Autodesk Fusion 360 part; units mm, degrees
sketch "Sketch1" plane through (0, 0, 0) normal (0, 0, 1) x (1, 0, 0)
  line L0 (0, 0) -> (-25, 0)
  line L1 (-25, 0) -> (-25, 25)
  line L2 (-25, 25) -> (0, 25)
  line L3 (0, 25) -> (0, 0)
  dimension "d1" = 25
  dimension "d2" = 25
extrude "Extrude1" add sketch "Sketch1" along normal blind 5
sketch "Sketch2" plane through (0, 0, 5) normal (0, 0, 1) x (-1, 0, 0)
  line L0 (0, -25) -> (25, -25)
  line L1 (25, -25) -> (25, 0)
  line L2 (25, 0) -> (0, 0)
  line L3 (0, 0) -> (0, -25)
  line L4 (12.5, -25) -> (12.5, 0)
  line L5 (12.5, -12.5) -> (0, -12.5)
  circle A0 centre (12.5, -12.5) radius 10
  dimension "d5" = 20
extrude "Extrude2" add sketch "Sketch2" along normal blind 5 contours L4 L5 A0 | L4 A0 | L4 L5 A0
sketch "Sketch3" plane through (0, 0, 10) normal (0, 0, 1) x (-1, 0, 0)
  circle A0 centre (12.5, -12.5) radius 10
  line L0 (11, -17) -> (14, -17)
  line L1 (14, -17) -> (14, -23)
  line L2 (14, -23) -> (11, -23)
  line L3 (11, -23) -> (11, -17)
extrude "Extrude3" cut sketch "Sketch3" against normal blind 3 contours A0 L0 L1 L3 picked at (12.6672, -18.8291)
Can you work these out from the model? Positions are in its coordinate system, mm. A direction names the side the tool comes from. Give positions to 0.01 mm unless a question says otherwise; leave off trailing zeros. Loops run counter-clockwise (first coordinate to the right, second up) from the corner with the lowest first, then second, coordinate; pieces in that order, holes last. Notation, with made-up numbers: M 56,88.25 L 77,88.25 A35 cw 77,126.25 Z; hole C -11.5,-35 d2. An arc over 180 degrees is marked long. Answer in a Markdown table with one row per item.
1. Suppose I cut it at B-B on x = -5.5. Write out the boundary of the cut face in (y, z).
Taken from the geometry:
| item | result |
|---|---|
| outline | M 0,0 L 25,0 L 25,5 L 19.64,5 L 19.64,10 L 5.36,10 L 5.36,5 L 0,5 Z |
2. Suppose I cut it at D-D on x = -12.5. Write out the boundary of the cut face in (y, z), plus the area to 4 significant figures.
Taken from the geometry:
| item | result |
|---|---|
| outline | M 0,0 L 25,0 L 25,5 L 22.5,5 L 22.5,7 L 17,7 L 17,10 L 2.5,10 L 2.5,5 L 0,5 Z |
| area | 208.5 mm² |
3. If I drill on line 1 along Z through (x, y) = (-19.25, 23.25); line 2 along X through (y, z) = (12.75, 8); line 3 along Y through (x, z) = (-18.5, 8), over which ranges is the centre line in solid material (lowest first)?
Taken from the geometry:
| item | result |
|---|---|
| line 1 | z = 0 to 5 |
| line 2 | x = -22.5 to -2.5 |
| line 3 | y = 4.5 to 20.5 |
4. Which directions (+Z, -Z, +X, -X, +Y, -Y) give clear straight access to the entire face, cutting with the end or side of a thin tool? Please do faces 5 (the flat face through (-13, 25, 2)), 6 (the flat face through (-12, 20, 7)), 7 (the flat face through (-21, 18.2, 5)).
Taken from the geometry:
| item | result |
|---|---|
| face 5 | +Z, -Z, +X, -X, +Y |
| face 6 | +Z, +Y |
| face 7 | +Z |
5. Suppose I cut it at C-C on z = 9.25. Write out the boundary of the cut face in (x, y), plus the area to 3 significant figures.
Taken from the geometry:
| item | result |
|---|---|
| outline | M -14,17 L -14,22.39 A10 ccw long -11,22.39 L -11,17 Z |
| area | 298 mm² |
6. Suppose I cut it at A-A on y = 12.5. Write out the boundary of the cut face in (x, z).
Taken from the geometry:
| item | result |
|---|---|
| outline | M -25,0 L 0,0 L 0,5 L -2.5,5 L -2.5,10 L -22.5,10 L -22.5,5 L -25,5 Z |
7. Thinking about a two-plate mould opening in X: for faces 1 (the flat face through (-25, 12, 2)), 2 (the flat face through (-12, 17, 9)), 3 (the flat face through (-12, 0, 2)), 4 (the flat face through (-11, 20, 9)), which applies, released by +X, released by -X, zero draft, split by the parting line, or undercut?
Taken from the geometry:
| item | result |
|---|---|
| face 1 | released by -X |
| face 2 | undercut |
| face 3 | zero draft |
| face 4 | undercut |
8. For pin 1 Ø2 at (x, z) = (-16, 7) entering from +Y; pin 2 Ø0.9 at (y, z) = (19, 9) entering from -X; pin 3 Ø0.9 at (y, z) = (19.5, 8.5) entering from +X, each with a flat end and sliding along its axis, tell me the tip position at first contact or that it passes through.
Taken from the geometry:
| item | result |
|---|---|
| pin 1 | stops at y = 22.18 |
| pin 2 | stops at x = -20.46 |
| pin 3 | stops at x = -4.94 |
